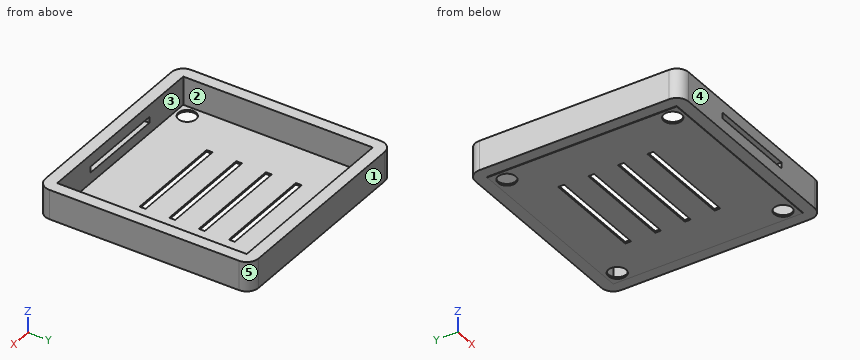
Autodesk Fusion 360 part; units mm, degrees
sketch "Sketch1" plane through (0, 0, 0) normal (0, 0, 1) x (1, 0, 0)
  line L0 (-27.6043, 30) -> (8.3957, 30)
  line L1 (8.3957, 30) -> (8.3957, -6)
  line L2 (8.3957, -6) -> (-27.6043, -6)
  line L3 (-27.6043, -6) -> (-27.6043, 30)
  line L4 (-25.6043, 28) -> (6.3957, 28)
  line L5 (6.3957, 28) -> (6.3957, -4)
  line L6 (6.3957, -4) -> (-25.6043, -4)
  line L7 (-25.6043, -4) -> (-25.6043, 28)
  dimension "d1" = 36
  dimension "d2" = 36
  dimension "d3" = 32
  dimension "d4" = 32
  dimension "d5" = 2
  dimension "d6" = 2
extrude "Extrude1" add sketch "Sketch1" along normal blind 5 from surface at 2 makes body 1
sketch "Sketch2" plane through (0, 0, 2) normal (0, 0, -1) x (1, 0, 0)
  line L0 (-25.6043, 4) -> (6.3957, 4)
  line L1 (6.3957, 4) -> (6.3957, -28)
  line L2 (6.3957, -28) -> (-25.6043, -28)
  line L3 (-25.6043, -28) -> (-25.6043, 4)
  line L4 (8.3957, 6) -> (-27.6043, 6)
  line L5 (-27.6043, 6) -> (-27.6043, -30)
  line L6 (-27.6043, -30) -> (8.3957, -30)
  line L7 (8.3957, -30) -> (8.3957, 6)
extrude "Extrude2" add sketch "Sketch2" along normal blind 0.2 separate body contours L0 L1 L2 L3 makes body 2
move_body "Move1" bodies 2 to x (1, 0, 0) y (0, 1, 0) z (0, 0, 1) at (0, 0, 0.2)
fillet "Fillet1" radius 2 1 edges at (-27.6043, 30, 4.5) on bodies 1
fillet "Fillet2" radius 2 1 edges at (-27.6043, -6, 4.5) on bodies 1
fillet "Fillet3" radius 2 1 edges at (8.3957, -6, 4.5) on bodies 1
fillet "Fillet4" radius 2 1 edges at (8.3957, 30, 4.5) on bodies 1
extrude "Extrude3" add 1 faces at (-14.9376, 17.3333, 2) along direction (0, 0, -1) blind 0.1 on bodies 2 bodies 1 2
sketch "Sketch3" plane through (0, 0, 2.2) normal (0, 0, 1) x (-1, 0, 0)
  line L0 (-6.3957, -28) -> (25.6043, -28)
  line L1 (25.6043, -28) -> (25.6043, 4)
  line L2 (25.6043, 4) -> (-6.3957, 4)
  line L3 (-6.3957, 4) -> (-6.3957, -28)
  circle A0 centre (23.6043, 2) radius 1.5
  circle A1 centre (23.6043, 2) radius 2
  circle A2 centre (-4.3957, 2) radius 1.5
  circle A3 centre (-4.3957, 2) radius 2
  circle A4 centre (-4.3957, -26) radius 1.5
  circle A5 centre (-4.3957, -26) radius 2
  circle A6 centre (23.6043, -26) radius 1.5
  circle A7 centre (23.6043, -26) radius 2
  dimension "d22" = 3
  dimension "d23" = 4
  dimension "d24" = 3
  dimension "d25" = 4
  dimension "d26" = 3
  dimension "d27" = 4
  dimension "d28" = 3
  dimension "d29" = 4
extrude "Extrude4" cut sketch "Sketch3" against normal blind 0.4 contours A2 bodies 1
extrude "Extrude5" cut sketch "Sketch3" against normal blind 4 contours A0 bodies 1
extrude "Extrude6" cut sketch "Sketch3" against normal blind 4 contours A6 bodies 1
extrude "Extrude7" cut sketch "Sketch3" against normal blind 4 contours A4 bodies 1
sketch "Sketch4" plane through (0, -6, 0) normal (0, -1, 0) x (1, 0, 0)
  line L0 (6.3957, 2) -> (6.3957, 7)
  line L1 (6.3957, 7) -> (-25.6043, 7)
  line L2 (-25.6043, 7) -> (-25.6043, 2)
  line L3 (-25.6043, 2) -> (6.3957, 2)
  line L4 (-17, 5) -> (-2, 5)
  line L5 (-2, 5) -> (-2, 4)
  line L6 (-2, 4) -> (-17, 4)
  line L7 (-17, 4) -> (-17, 5)
extrude "Extrude8" cut sketch "Sketch4" against normal blind 5 contours L4 L5 L6 L7 bodies 1
sketch "Sketch5" plane through (0, 0, 2.2) normal (0, 0, 1) x (-1, 0, 0)
  circle A0 centre (-4.3957, -26) radius 1.5
  circle A1 centre (23.6043, -26) radius 1.5
  circle A2 centre (23.6043, 2) radius 1.5
  circle A3 centre (-4.3957, 2) radius 1.5
  line L0 (-6.3957, -28) -> (25.6043, -28)
  line L1 (25.6043, -28) -> (25.6043, 4)
  line L2 (25.6043, 4) -> (-6.3957, 4)
  line L3 (-6.3957, 4) -> (-6.3957, -28)
  line L4 (18, -16) -> (1, -16)
  line L5 (1, -16) -> (1, -15)
  line L6 (1, -15) -> (18, -15)
  line L7 (18, -15) -> (18, -16)
  line L8 (1, -11) -> (18, -11)
  line L9 (18, -11) -> (18, -10)
  line L10 (18, -10) -> (1, -10)
  line L11 (1, -10) -> (1, -11)
  line L12 (18, -6) -> (1, -6)
  line L13 (1, -6) -> (1, -5)
  line L14 (1, -5) -> (18, -5)
  line L15 (18, -5) -> (18, -6)
  line L16 (18.1043, -21) -> (1.1043, -21)
  line L17 (1.1043, -21) -> (1.1043, -20)
  line L18 (1.1043, -20) -> (18.1043, -20)
  line L19 (18.1043, -20) -> (18.1043, -21)
  dimension "d40" = 7
  dimension "d41" = 7.5
  dimension "d42" = 4
  dimension "d43" = 4
  dimension "d44" = 4
extrude "Extrude9" cut sketch "Sketch5" against normal blind 5 contours L16 L17 L18 L19 bodies 1
extrude "Extrude10" cut sketch "Sketch5" against normal blind 5 contours L4 L5 L6 L7 | L8 L9 L10 L11 | L12 L13 L14 L15 bodies 1
Model file for the job. Use its own axes, mm. Face numbers are marked on the shaded views. A direction names the side the tool comes from. Coordinates: 2 decimals unless noted, no trailing zeros. Loops run counter-clockwise (first coordinate to the right, second up) from the corner with the lowest first, then second, coordinate; pieces in that order, holes last. Notation, with made-up numbers: M 39.25,49 L 92.25,49 A17 ccw 92.25,56 Z; hole C -35,-6 d4. An arc over 180 degrees is marked long. Use CSV: the item, a comma, the result in double quotes. Start each with the question number.
1. Band-saw the part on B-B, the plane x = -3. Give the number of separate pieces and of enclosed holes in the cut face, then the cut area to 3 significant figures.
2. Probe probe 1 along X at (y, z) = (26, 2.15); probe 2 along Y at (x, z) = (4, 3.9); probe 3 along X at (y, z) = (10, 3.85). List the from-to ranges inside material, lowest first. Write a range as [from, to].
3. Band-saw the part on A-A, the plane y = -2. List the corners of the cut face in (x, z), then the cut area to 3 significant figures.
4. Flat gauge pins, fed straight in: pin 1 (0.8 mm diameter, centred on y = -4.5, z = 4.5, fed in from +X); pin 2 (8 mm diameter, centred on x = -21.5, y = 2.5, fed in from +Z). Where does each tip first touch, or does it go through?
5. Two-plate mould, pull along Y, no slides. Class the marked faces 3, 4 and 5: pulls with the +Y half, pulls with the -Y half, needs draft (parallel to the pull), parting line crosses it, or undercut.
6. Band-saw the part on C-C, the plane z = 6.45. List the corners of the cut face in (x, y).
7. Tool access for the marked faces 1 and 2: list every direction of +Z, -Z, +X, -X, +Y, -Y with a clear straight run to the whole face (end or side of a thin tool).
8. Band-saw the part on D-D, the plane x = 1. List the corners of the cut face in (y, z), then the cut area to 3 significant figures.
Entries:
1,separate pieces,"6"
1,enclosed holes,"0"
1,area,"26.4 mm2"
2,probe 1,"x = [-27.6, -25.1], [-22.1, 2.9], [5.9, 8.4]"
2,probe 2,"y = [-6, -4], [28, 30]"
2,probe 3,"x = [-27.6, -25.6], [6.4, 8.4]"
3,outline,"M -27.6,2 L -25.6,2 L -25.6,1.9 L -25.1,1.9 L -25.1,2.2 L -25.6,2.2 L -25.6,7 L -27.6,7 Z; M -22.1,1.9 L 2.9,1.9 L 2.9,2.2 L -22.1,2.2 Z; M 5.9,1.9 L 6.4,1.9 L 6.4,2 L 8.4,2 L 8.4,7 L 6.4,7 L 6.4,2.2 L 5.9,2.2 Z"
3,area,"27.8 mm2"
4,pin 1,"stops at x = 8.39"
4,pin 2,"stops at z = 2.2"
5,face 3,"undercut"
5,face 4,"pulls with the -Y half"
5,face 5,"pulls with the +Y half"
6,outline,"M -27.6,-4 A2 ccw -25.6,-6 L 6.4,-6 A2 ccw 8.4,-4 L 8.4,28 A2 ccw 6.4,30 L -25.6,30 A2 ccw -27.6,28 Z; hole M -25.6,-4 L 6.4,-4 L 6.4,28 L -25.6,28 Z"
7,face 1,"+Z, -Z, +X, -X, +Y"
7,face 2,"+Z"
8,outline,"M -6,2 L -4,2 L -4,1.9 L 28,1.9 L 28,2 L 30,2 L 30,7 L 28,7 L 28,2.2 L -4,2.2 L -4,7 L -6,7 Z"
8,area,"29.6 mm2"
